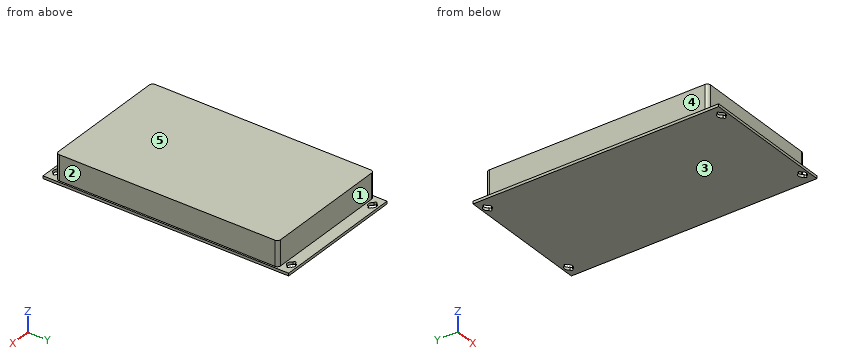
Autodesk Inventor part; units mm, degrees
ref_plane "YZ Plane" through (0, 0, 0) normal (1, 0, 0) x (0, 1, 0)
ref_plane "XZ Plane" through (0, 0, 0) normal (0, 1, 0) x (-1, 0, 0)
ref_plane "XY Plane" through (0, 0, 0) normal (0, 0, 1) x (1, 0, 0)
sketch "Sketch1" plane through (0, 0, 0) normal (0, 0, 1) x (1, 0, 0)
  line L0 (40, 73.5) -> (-40, 73.5)
  line L1 (-40, 73.5) -> (-40, -73.5)
  line L2 (-40, -73.5) -> (40, -73.5)
  line L3 (40, -73.5) -> (40, 73.5)
  line L4 (40, 73.5) -> (-40, -73.5) construction
  line L5 (-40, 73.5) -> (40, -73.5) construction
  line L6 (-33, 70) -> (33, 70) construction
  line L7 (33, 70) -> (33, -70) construction
  line L8 (33, -70) -> (-33, -70) construction
  line L9 (-33, -70) -> (-33, 70) construction
  line L10 (-33, 70) -> (33, -70) construction
  line L11 (33, 70) -> (-33, -70) construction
  line L12 (40, 0) -> (-40, 0) construction
  line L13 (0, 73.5) -> (0, -73.5) construction
  circle A0 centre (33, 70) radius 2.4
  circle A1 centre (-33, 70) radius 2.4
  circle A2 centre (33, -70) radius 2.4
  circle A3 centre (-33, -70) radius 2.4
  line L14 (33, 73.25) -> (33, 66.75) construction
  arc A4 (35.2895, 69.2801) -> (35.2895, 70.7199) centre (35.5, 70) ccw
  arc A5 (30.7105, 70.7199) -> (30.7105, 69.2801) centre (30.5, 70) ccw
  arc A6 (-35.2895, 70.7199) -> (-35.2895, 69.2801) centre (-35.5, 70) ccw
  arc A7 (-30.7105, 69.2801) -> (-30.7105, 70.7199) centre (-30.5, 70) ccw
  arc A8 (35.2895, -70.7199) -> (35.2895, -69.2801) centre (35.5, -70) ccw
  arc A9 (30.7105, -69.2801) -> (30.7105, -70.7199) centre (30.5, -70) ccw
  arc A10 (-35.2895, -69.2801) -> (-35.2895, -70.7199) centre (-35.5, -70) ccw
  arc A11 (-30.7105, -70.7199) -> (-30.7105, -69.2801) centre (-30.5, -70) ccw
  line L15 (39, 66.5) -> (-39, 66.5)
  line L16 (-39, 66.5) -> (-39, -66.5)
  line L17 (-39, -66.5) -> (39, -66.5)
  line L18 (39, -66.5) -> (39, 66.5)
  line L19 (39, 66.5) -> (-39, -66.5) construction
  line L20 (-39, 66.5) -> (39, -66.5) construction
  point P0 (0, 0)
  point P1 (36.25, 70)
  point P2 (29.75, 70)
  point P3 (36.25, -70)
  point P4 (30.7105, 69.2801)
  point P5 (30.7105, 70.7199)
  point P6 (-30.7105, 70.7199)
  point P7 (-30.7105, 69.2801)
  point P8 (-35.2895, 69.2801)
  point P9 (-35.2895, 70.7199)
  point P10 (-30.7105, -69.2801)
  point P11 (-30.7105, -70.7199)
  point P12 (-35.2895, -70.7199)
  point P13 (-35.2895, -69.2801)
  point P14 (35.2895, -69.2801)
  point P15 (35.2895, -70.7199)
  point P16 (30.7105, -70.7199)
  point P17 (30.7105, -69.2801)
  dimension "d0" = 80
  dimension "d1" = 147
  dimension "d19" = 4.8
  dimension "d30" = 6.5
  dimension "d33" = 140
  dimension "d34" = 66
  dimension "d35" = 6.5
  dimension "d36" = 1.5
  dimension "d37" = 7
  dimension "d38" = 1
  dimension "d39" = 133
  dimension "d40" = 78
  dimension "d41" = 14
extrude "Extrusion1" add sketch "Sketch1" along normal blind 1.6 contours L3 L2 L1 L0 | L18 L17 L16 L15
extrude "Extrusion2" add sketch "Sketch1" along normal blind 16.6 contours L18 L17 L16 L15
fillet "Fillet1" radius 2 4 edges at (39, -66.5, 9.1) (39, 66.5, 9.1) (-39, -66.5, 9.1) (-39, 66.5, 9.1)
properties part number "SUSTAINA-POWER-MONITOR-BOARD" material "Acetal Resin, Black"
Build history of the part. All positions in model axes, mm. Face numbers are marked on the shaded views. A direction names the side the tool comes from. Round coordinates to 2 decimals unless told otherwise and drop trailing zeros. Write each loop counter-clockwise with the first axis right and the second up, starting at its lowest first coordinate (ties: lowest second). Pieces come first, ordered by that corner, then holes. Notation, with made-up numbers: (74.25, -7.5) - (84.25, -7.5) arc R23 ccw to (84.25, 31.5) - close; hole circle Ø4 at (-26.5, 35.5). An arc over 180 degrees is marked (long way). Answer as CSV lines item,"result".
Q1. Drop flat-ended pins along their axis: pin 1 (1 mm diameter, centred on x = -26, z = 11, fed in from +Y); pin 2 (8 mm diameter, centred on y = 18.5, z = 14, fed in from -X); pin 3 (1.4 mm diameter, centred on x = -35.5, y = 70, fed in from -Z); pin 4 (1.7 mm diameter, centred on x = 35.5, y = 70, fed in from +Z). Give the stop position or say it passes through.
Report:
pin 1,"stops at y = 66.5"
pin 2,"stops at x = -39"
pin 3,"passes through"
pin 4,"stops at z = 1.6"
Q2. Tool access for the marked faces 1, 2, 3, 4 and 5: list every direction of +Z, -Z, +X, -X, +Y, -Y with a clear straight run to the whole face (end or side of a thin tool).
Report:
face 1,"+Z, +X, -X, +Y"
face 2,"+Z, +X, +Y, -Y"
face 3,"-Z, +X, -X, +Y, -Y"
face 4,"+Z, -X, +Y, -Y"
face 5,"+Z, +X, -X, +Y, -Y"
Q3. Cut at A-A (y = 11). Write the cut outline in (x, z).
Report:
outline,"(-40, 0) - (40, 0) - (40, 1.6) - (39, 1.6) - (39, 16.6) - (-39, 16.6) - (-39, 1.6) - (-40, 1.6) - close"
Q4. Drill centre lines: probe 1 along Y at (x, z) = (-30.5, 0.4); probe 2 along Y at (x, z) = (-27.5, 14.75); probe 3 along X at (y, z) = (58.5, 8.75). Where is each one in solid material? Low to high. Write a range as [from, to].
Report:
probe 1,"y = [-73.5, -70.75], [-69.25, 69.25], [70.75, 73.5]"
probe 2,"y = [-66.5, 66.5]"
probe 3,"x = [-39, 39]"
Q5. Cut at B-B (z = 4). Write the cut outline in (x, y), and give its area (3 significant figures).
Report:
outline,"(-39, -64.5) arc R2 ccw to (-37, -66.5) - (37, -66.5) arc R2 ccw to (39, -64.5) - (39, 64.5) arc R2 ccw to (37, 66.5) - (-37, 66.5) arc R2 ccw to (-39, 64.5) - close"
area,"10,400 mm^2"
